Geometry check sheet. Reference: the model listing, model coordinates, mm. A direction names the side the tool comes from. Round coordinates to 2 decimals unless told otherwise and drop trailing zeros. Loops run counter-clockwise (first coordinate to the right, second up) from the corner with the lowest first, then second, coordinate; pieces in that order, holes last. Notation, with made-up numbers: (40, 50) - (78, 50) arc R32 cw to (78, 85) - close; hole circle Ø4 at (49.25, 34.5). An arc over 180 degrees is marked (long way). Answer as CSV lines item,"result". Start each with the question number.
1) Thickness scan on line 1 along Y through (x, z) = (0, 20); line 2 along Z through (x, y) = (0, -3.5); line 3 along X through (y, z) = (-2, 0). Record the ranges inside material, lowest first.
2) Depth check by flat-ended pin: P1, Ø6, axis at x = -16, z = -6, coming from the -Y side; P2, Ø1.5, axis at y = -3.5, z = 21, coming from the +X side; P3, Ø5.5, axis at y = -7, z = 22.5, coming from the -X side; P4, Ø6, axis at y = -4, z = 10.5, coming from the -X side. Enter the tip coordinate at first touch or a pass-through.
3) Cross-section at B-B on y = -7.5. Record the boundary of the cut face in (x, z).
4) Access from +Z, -Z, +X, -X, +Y, -Y to the whole of each face (thin tool, end or side, straight path). Record for faces 1 (the flat face through (-4.202, -5, 22)), 2 (the flat face through (3.919, -5, 22)), 3 (the flat face through (0, -5, 18.547)), 4 (the flat face through (9.93, -4.93, 16.06)).
5) Cross-section at C-C on z = 0. Record the boundary of the cut face in (x, y), and give its area (3 significant figures).
6) Cross-section at A-A on x = 0. Record the boundary of the cut face in (y, z), and give its area (3 significant figures).
7) Draft check along X on faces 5 (the flat face through (12, -4.93, -14.62)), 6 (the cylindrical face through (0.62, -6.2, 21.59)), 7 (the flat face through (-1, -3.8, 24.547)). Enter one of: released by +X, released by -X, zero draft, split by the parting line, or undercut.
8) Cross-section at D-D on y = -5. Record the boundary of the cut face in (x, z), and give its area (3 significant figures).
from build123d import *

# Parameters (mm, degrees)
F1_DEPTH = 10
F2_R     = 1.35
F3_DEPTH = 6


with BuildPart() as f1:
    # F0 (on Front) → F1 (new body)
    with BuildSketch(Plane.XZ):
        with BuildLine():
            ThreePointArc((11.34649, -13.844391), (-17.859135, -1.208842), (9.377353, 15.247139))
            Line((9.377353, 15.247139), (10.500295, 16.904254))
            ThreePointArc((10.500295, 16.904254), (7.326353, 18.502285), (3.918794, 19.510332))
            Line((3.918794, 19.510332), (3.918794, 24.546802))
            Line((3.918794, 24.546802), (-4.201883, 24.546802))
            Line((-4.201883, 24.546802), (-4.201883, 19.451328))
            ThreePointArc((-4.201883, 19.451328), (-17.915323, -8.663209), (12.63751, -15.372161))
            Line((12.63751, -15.372161), (11.34649, -13.844391))
        make_face()
    extrude(amount=F1_DEPTH)

    # F2 (on face) → F3 (cut)
    with BuildSketch(Plane.XY.offset(24.546802)):
        with Locations((0, -5)):
            Circle(F2_R)
    extrude(amount=-F3_DEPTH, mode=Mode.SUBTRACT)


solid = f1.part
Answer block:
1,line 1,"y = -10 to -6.35, -3.65 to 0"
1,line 2,"z = -19.9 to -17.9, 17.9 to 24.55"
1,line 3,"x = -19.9 to -17.9"
2,P1,"stops at y = -10"
2,P2,"stops at x = 3.92"
2,P3,"stops at x = -4.2"
2,P4,"stops at x = -18.43"
3,outline,"(-4.2, 19.45) arc R19.9 ccw (long way) to (12.64, -15.37) - (11.35, -13.84) arc R17.9 cw (long way) to (9.38, 15.25) - (10.5, 16.9) arc R19.9 ccw to (3.92, 19.51) - (3.92, 24.55) - (-4.2, 24.55) - close"
4,face 1,"+Z, -X, +Y, -Y"
4,face 2,"+Z, +X, +Y, -Y"
4,face 3,"+Z"
4,face 4,"+X, +Y, -Y"
5,outline,"(-19.9, -10) - (-17.9, -10) - (-17.9, 0) - (-19.9, 0) - close"
5,area,"20.0 mm^2"
6,outline,"(-10, -19.9) - (0, -19.9) - (0, -17.9) - (-10, -17.9) - close; (-10, 17.9) - (0, 17.9) - (0, 24.55) - (-3.65, 24.55) - (-3.65, 18.55) - (-6.35, 18.55) - (-6.35, 24.55) - (-10, 24.55) - close"
6,area,"70.3 mm^2"
7,face 5,"released by +X"
7,face 6,"undercut"
7,face 7,"zero draft"
8,outline,"(-4.2, 19.45) arc R19.9 ccw (long way) to (12.64, -15.37) - (11.35, -13.84) arc R17.9 cw (long way) to (9.38, 15.25) - (10.5, 16.9) arc R19.9 ccw to (3.92, 19.51) - (3.92, 24.55) - (1.35, 24.55) - (1.35, 18.55) - (-1.35, 18.55) - (-1.35, 24.55) - (-4.2, 24.55) - close"
8,area,"188 mm^2"
